Could you check a few things on this model? Use its own coordinates, in mm. Coordinates: 2 decimals unless noted, no trailing zeros. Loops run counter-clockwise (first coordinate to the right, second up) from the corner with the lowest first, then second, coordinate; pieces in that order, holes last. Notation, with made-up numbers: (31.25, 61.25) - (45.25, 61.25) arc R31 cw to (45.25, 98.25) - close; hole circle Ø9 at (-22, 29.5). An arc over 180 degrees is marked (long way). One line per question, with ' | ' between items. Start each with the question number.
1. I'm going to push flat-ended pins straight in: P1, Ø0.9, axis at x = 497, z = 1, coming from the -Y side; P2, Ø1, axis at y = 90.5, z = 2, coming from the +X side; P3, Ø1, axis at y = 53, z = 2.5, coming from the -X side. Where does each tip first touch, or does it pass through?
2. I want a section at D-D, the plane x = 499.5. Write out the boundary of the cut face in (y, z).
3. I want a section at C-C, the plane z = 0.75. Write out the boundary of the cut face in (x, y).
4. I want a section at A-A, the plane y = 78.5. Write out the boundary of the cut face in (x, z).
5. Please list where these lines run through material, in increasing order: L1, parallel to Y at x = 496.5, z = 1.95; L2, parallel to Y at x = 495.25, z = 1.3; L3, parallel to X at y = 74.5, z = 0.65. Write a range as [from, to].
6. I want a section at B-B, the plane x = 497.25. Write out the boundary of the cut face in (y, z), then the cut area to 3 significant figures.
from build123d import *

# Parameters (mm, degrees)
SKETCH1_W          = 3
SKETCH1_H          = 20
BASE_EXTRUDE_DEPTH = 3


with BuildPart() as part:
    # Sketch1 → Base-Extrude (new body)
    with BuildSketch(Plane.XY):
        with BuildLine():
            Line((490.859334316, 48.711445231), (490.859334316, 91.178595635))
            ThreePointArc((490.859334316, 91.178595635), (492.980510735, 97.046258165), (498.958835763, 98.831890501))
            ThreePointArc((498.958835763, 98.831890501), (499.873560394, 98.672316261), (500.789492391, 98.519824725))
            ThreePointArc((500.789492391, 98.519824725), (507.814480551, 95.282897305), (512.167074898, 88.888909486))
            ThreePointArc((512.167074898, 88.888909486), (510.632309562, 66.803543283), (502.248398483, 46.313815613))
            ThreePointArc((502.248398483, 46.313815613), (499.455679175, 43.623308538), (495.646031752, 42.898949534))
            ThreePointArc((495.646031752, 42.898949534), (494.9563895, 47.208231088), (490.859334316, 48.711445231))
        make_face()
        with Locations((496.503228356, 72.313930056)):
            Rectangle(SKETCH1_W, SKETCH1_H, mode=Mode.SUBTRACT)
    extrude(amount=BASE_EXTRUDE_DEPTH)


solid = part.part
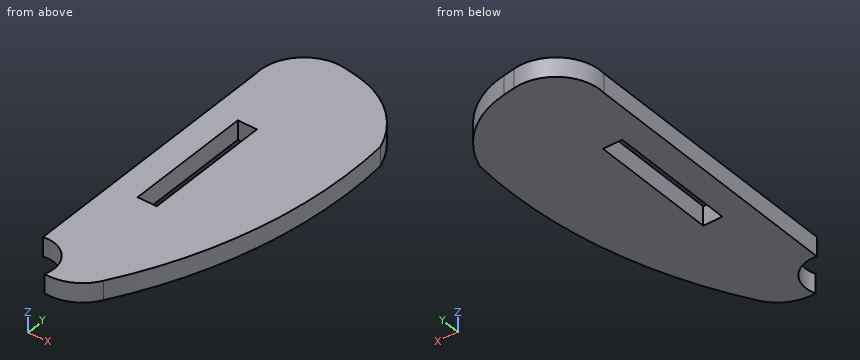
Results are:
1) P1: stops at y = 42.87 | P2: stops at x = 511.74 | P3: stops at x = 490.86
2) outline: (43.65, 0) - (98.74, 0) - (98.74, 3) - (43.65, 3) - close
3) outline: (490.86, 48.71) arc R4.31 cw to (495.65, 42.9) arc R6.79 ccw to (502.25, 46.31) arc R69.69 ccw to (512.17, 88.89) arc R14.46 ccw to (500.79, 98.52) arc R120 cw to (498.96, 98.83) arc R6.93 ccw to (490.86, 91.18) - close; hole (495, 62.31) - (498, 62.31) - (498, 82.31) - (495, 82.31) - close
4) outline: (490.86, 0) - (495, 0) - (495, 3) - (490.86, 3) - close; (498, 0) - (512.33, 0) - (512.33, 3) - (498, 3) - close
5) L1: y = [42.87, 62.31], [82.31, 98.83] | L2: y = [46.81, 62.31], [82.31, 98.48] | L3: x = [490.86, 495], [498, 511.98]
6) outline: (42.93, 0) - (62.31, 0) - (62.31, 3) - (42.93, 3) - close; (82.31, 0) - (98.92, 0) - (98.92, 3) - (82.31, 3) - close | area: 108 mm2
